Input: part model. Units: mm. Frame: model coordinates. Round coordinates to 2 decimals unless told otherwise and drop trailing zeros. Loops run counter-clockwise (first coordinate to the right, second up) from the corner with the lowest first, then second, coordinate; pieces in that order, holes last. Notation, with made-up numbers: (-37.75, 36) -> (6.25, 36) arc R23 cw to (6.25, 60) -> close; hole circle Ø4 at (28.5, 14.25). An arc over 180 degrees is marked (long way). One line per question, with ' | ' between items. Start each with the question number.
Q1. Cut plane A-A on z = 97. Return loops of the section in (x, y), and give its area (3 significant figures).
Q2. Material intervals for L1, parallel to Z at x = 5, y = 21; L2, parallel to X at y = 15.5, z = 28.5; L3, parallel to X at y = 14.5, z = 557.5, sorted ascending.
Q3. Contact query for flat-ended pins moving along their axis: P1, Ø4, axis at y = -8, z = 262.5, coming from the +X side; P2, Ø6, axis at y = 1.5, z = 376.5, coming from the -X side; P3, Ø10, axis at x = 13.5, z = 318.5, coming from the +Y side; P4, Ø25, axis at x = -8.5, y = -11.5, coming from the +Z side. Output: stop coordinate, or through.
from build123d import *

# Parameters (mm, degrees)
SKETCH1_R           = 25.4
BOSS_EXTRUDE1_DEPTH = 590.55
SKETCH2_OUTSIDE_W   = 171.78
SKETCH2_OUTSIDE_H   = 171.78
SKETCH2_OUTSIDE_R   = 6.361935525
CUT_EXTRUDE1_DEPTH  = 25.4
SKETCH5_OUTSIDE_W   = 171.78
SKETCH5_OUTSIDE_H   = 171.78
SKETCH5_OUTSIDE_R   = 6.377907631
CUT_EXTRUDE4_DEPTH  = 25.4
CUT_EXTRUDE5_DEPTH  = 568.96
CIRPATTERN1_COUNT   = 4


with BuildPart() as part:
    # Sketch1 → Boss-Extrude1 (new body)
    with BuildSketch(Plane.XY):
        Circle(SKETCH1_R)
    extrude(amount=BOSS_EXTRUDE1_DEPTH)

    # Sketch2 outside → Cut-Extrude1 (cut)
    with BuildSketch(Plane.XY):
        Rectangle(SKETCH2_OUTSIDE_W, SKETCH2_OUTSIDE_H)
        Circle(SKETCH2_OUTSIDE_R, mode=Mode.SUBTRACT)
    extrude(amount=CUT_EXTRUDE1_DEPTH, mode=Mode.SUBTRACT)

    # Sketch5 outside → Cut-Extrude4 (cut)
    with BuildSketch(Plane.XY.offset(590.55)):
        Rectangle(SKETCH5_OUTSIDE_W, SKETCH5_OUTSIDE_H)
        Circle(SKETCH5_OUTSIDE_R, mode=Mode.SUBTRACT)
    extrude(amount=-CUT_EXTRUDE4_DEPTH, mode=Mode.SUBTRACT)

    # Sketch6 → Cut-Extrude5 (cut)
    with BuildSketch(Plane.XY):
        with BuildLine():
            ThreePointArc((29.164386469, 0), (26.85091062, 11.383761989), (20.277517743, 20.961481635))
            ThreePointArc((20.277517743, 20.961481635), (14.954603392, 20.873199153), (15.042885874, 15.550284802))
            ThreePointArc((15.042885874, 15.550284802), (19.919360406, 8.445049073), (21.635613531, 0))
            ThreePointArc((21.635613531, 0), (25.4, -3.764386469), (29.164386469, 0))
        make_face()
    cut_extrude5 = extrude(amount=CUT_EXTRUDE5_DEPTH, mode=Mode.SUBTRACT)

    # CirPattern1: Cut-Extrude5 ×4 about axis
    cirpattern1_axis = Axis((0, 0, 0), (0, 0, 1))
    for i in range(1, CIRPATTERN1_COUNT):
        add(cut_extrude5.rotate(cirpattern1_axis, i * 360 / CIRPATTERN1_COUNT), mode=Mode.SUBTRACT)


solid = part.part
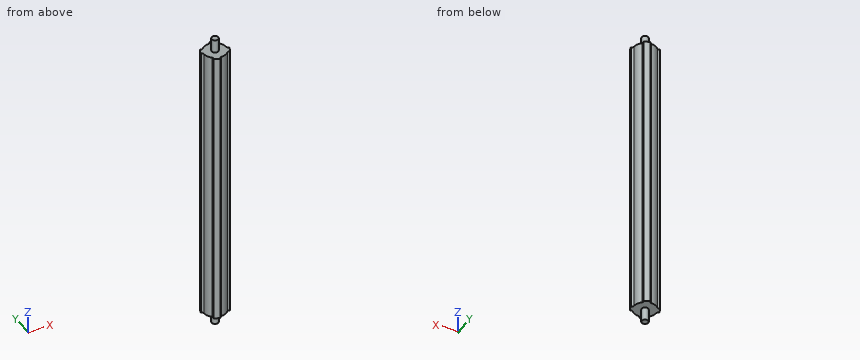
Results:
1) outline: (-25.12, 3.75) arc R3.76 cw to (-21.64, 0) arc R21.64 ccw to (-15.04, -15.55) arc R3.76 cw to (-14.77, -20.67) arc R25.4 ccw to (-3.75, -25.12) arc R3.76 cw to (0, -21.64) arc R21.64 ccw to (15.55, -15.04) arc R3.76 cw to (20.67, -14.77) arc R25.4 ccw to (25.12, -3.75) arc R3.76 cw to (21.64, 0) arc R21.64 ccw to (15.04, 15.55) arc R3.76 cw to (14.77, 20.67) arc R25.4 ccw to (3.75, 25.12) arc R3.76 cw to (0, 21.64) arc R21.64 ccw to (-15.55, 15.04) arc R3.76 cw to (-20.67, 14.77) arc R25.4 ccw to start | area: 1,660 mm^2
2) L1: 25.4 to 565.15 | L2: -15.09 to 15.09 | L3: -20.85 to -20.3, -16.21 to 16.06
3) P1: x = 24.68 | P2: x = -25.12 | P3: y = 23.94 | P4: z = 590.55
